from build123d import *

# Parameters (mm, degrees)
CROQUIS1_W              = 5
CROQUIS1_H              = 33
SALIENTE_EXTRUIR1_DEPTH = 3
CROQUIS3_W              = 7
CROQUIS3_H              = 3
SALIENTE_EXTRUIR2_DEPTH = 7
CORTAR_EXTRUIR1_REACH   = 75.478
CROQUIS4_W              = 4.98
CROQUIS4_H              = 6
CROQUIS5_R              = 1
CORTAR_EXTRUIR4_DEPTH   = 15
CORTAR_EXTRUIR5_DEPTH   = 15
CROQUIS8_W              = 2.5
CROQUIS8_H              = 4.326412588
CORTAR_EXTRUIR6_DEPTH   = 10
CORTAR_EXTRUIR7_REACH   = 75.146
CROQUIS9_W              = 1.2
CROQUIS9_H              = 27.63275501


with BuildPart() as part:
    # Croquis1 → Saliente-Extruir1 (new body)
    with BuildSketch(Plane.XY):
        with Locations((-8.507787801, 55.928529755)):
            Rectangle(CROQUIS1_W, CROQUIS1_H)
    extrude(amount=SALIENTE_EXTRUIR1_DEPTH)

    # Croquis3 → Saliente-Extruir2 (add)
    with BuildSketch(Plane.XZ.offset(-39.428529755)):
        with Locations((-8.507787801, 1.5)):
            Rectangle(CROQUIS3_W, CROQUIS3_H)
    extrude(amount=SALIENTE_EXTRUIR2_DEPTH)

    # Croquis4 → Cortar-Extruir1 (cut, up to next)
    with BuildSketch(Plane.XY.offset(3), mode=Mode.PRIVATE) as cortar_extruir1_sk1:
        with Locations((-8.507787801, 35.428529755)):
            Rectangle(CROQUIS4_W, CROQUIS4_H)
    cortar_extruir1_tool1 = extrude(cortar_extruir1_sk1.sketch, amount=-CORTAR_EXTRUIR1_REACH, mode=Mode.PRIVATE) & part.part
    add(cortar_extruir1_tool1.solids().sort_by_distance((-8.507788, 35.42853, 3))[0], mode=Mode.SUBTRACT)

    # Croquis5 → Cortar-Extruir4 (cut)
    with BuildSketch(Plane.ZY.offset(12.007787801)):
        with Locations(Location((1.5, 70.414414657, 0), (0, 0, 270))):
            Circle(CROQUIS5_R)
        with Locations((1.5, 34.917908979)):
            Circle(CROQUIS5_R)
    extrude(amount=-CORTAR_EXTRUIR4_DEPTH, mode=Mode.SUBTRACT)

    # Croquis7 → Cortar-Extruir5 (cut)
    with BuildSketch(Plane.ZY.offset(12.007787801)):
        with BuildLine():
            Line((3, 71.470870039), (3, 72.821585946))
            Line((3, 72.821585946), (0, 72.821585946))
            Line((0, 72.821585946), (0, 71.470870039))
            ThreePointArc((0, 71.470870039), (1.5, 72.091024013), (3, 71.470870039))
        make_face()
        with BuildLine():
            Line((0, 34.344024201), (0, 31.961571753))
            Line((0, 31.961571753), (3, 31.961571753))
            Line((3, 31.961571753), (3, 34.344024201))
            ThreePointArc((3, 34.344024201), (1.5, 33.311875437), (0, 34.344024201))
        make_face()
    extrude(amount=-CORTAR_EXTRUIR5_DEPTH, mode=Mode.SUBTRACT)

    # Croquis8 → Cortar-Extruir6 (cut)
    with BuildSketch(Plane.XY.offset(3)):
        with Locations((-8.507787801, 70.224491059)):
            Rectangle(CROQUIS8_W, CROQUIS8_H)
    extrude(amount=-CORTAR_EXTRUIR6_DEPTH, mode=Mode.SUBTRACT)

    # Croquis9 → Cortar-Extruir7 (cut, up to next)
    with BuildSketch(Plane.XY.offset(3), mode=Mode.PRIVATE) as cortar_extruir7_sk1:
        with Locations((-10.407787801, 53.24490726)):
            Rectangle(CROQUIS9_W, CROQUIS9_H)
    cortar_extruir7_tool1 = extrude(cortar_extruir7_sk1.sketch, amount=-CORTAR_EXTRUIR7_REACH, mode=Mode.PRIVATE) & part.part
    # Croquis9 → Cortar-Extruir7 (cut, up to next)
    with BuildSketch(Plane.XY.offset(3), mode=Mode.PRIVATE) as cortar_extruir7_sk2:
        with Locations((-6.607787801, 53.24490726)):
            Rectangle(CROQUIS9_W, CROQUIS9_H)
    cortar_extruir7_tool2 = extrude(cortar_extruir7_sk2.sketch, amount=-CORTAR_EXTRUIR7_REACH, mode=Mode.PRIVATE) & part.part
    add(cortar_extruir7_tool1.solids().sort_by_distance((-10.407788, 53.244907, 3))[0], mode=Mode.SUBTRACT)
    add(cortar_extruir7_tool2.solids().sort_by_distance((-6.607788, 53.244907, 3))[0], mode=Mode.SUBTRACT)


solid = part.part
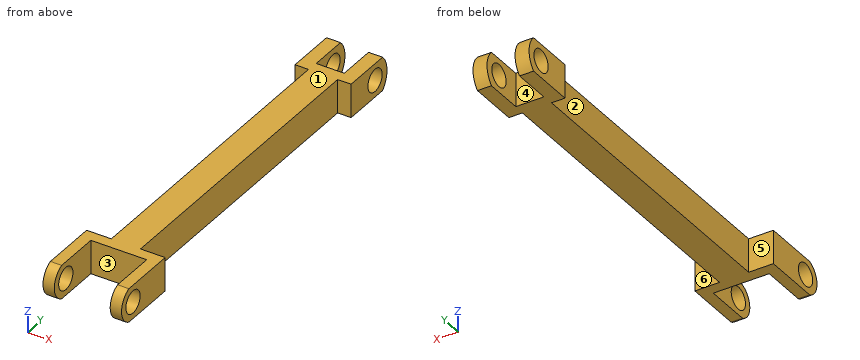
Here's how the part is built. I have some questions about the finished solid (model axes, mm). Face numbers are marked on the shaded views. A direction names the side the tool comes from. Give positions to 0.01 mm unless a question says otherwise; leave off trailing zeros. Write each loop counter-clockwise with the first axis right and the second up, starting at its lowest first coordinate (ties: lowest second). Pieces come first, ordered by that corner, then holes. Notation, with made-up numbers: (-12.5, 57) -> (-5.5, 57) arc R13 cw to (-5.5, 70) -> close; hole circle Ø9 at (11.5, 39). An arc over 180 degrees is marked (long way). Use one line per item in the form item = value. Start each with the question number.
1. Imagine slicing it at B-B on x = -10.5. List the corners of the cut face in (y, z) for me.
2. Imagine slicing it at D-D on x = -5.5. List the corners of the cut face in (y, z) for me.
3. Will these pins go through, and if not, where does the flat tip stop? pin 1 Ø1.3 at (x, z) = (-7, 1) entering from -Y; pin 2 Ø1 at (x, z) = (-8.5, 1.5) entering from +Y; pin 3 Ø1.5 at (y, z) = (69.5, 1) entering from -X.
4. On a 3-axis mill with a long thin cutter (end or side, diameter ignored), from which of +Z, -Z, +X, -X, +Y, -Y can I reach the whole of each face in a straight line? I mean the marked faces 4, 5 and 6. Say none if no direction works.
5. Imagine slicing it at A-A on y = 38. List the corners of the cut face in (x, z) for me.
6. Thinking about a two-plate mould opening in Y: for the marked faces 1, 2 and 3, which applies, +Y half, -Y half, draft (parallel to the pull), parting line (faces both ways), or undercut?
7. If I drill on L1, parallel to X at y = 68.5, z = 0.35; L2, parallel to X at y = 37.5, z = 1.5; L3, parallel to X at y = 46, z = 0.65, over which ranges is the centre line in solid material (lowest first)?
8. Imagine slicing it at C-C on z = 1.5. State how many separate pieces and enclosed holes the cut face has, plus the area to 3 significant figures.
Entries:
q1.outline = (38.43, 0) -> (39.43, 0) -> (39.43, 3) -> (38.43, 3) -> close; (67.06, 0) -> (71.47, 0) arc R2.12 ccw to (71.47, 3) -> (67.06, 3) -> close; hole circle Ø2 at (70.41, 1.5)
q2.outline = (34.34, 0) -> (39.43, 0) -> (39.43, 3) -> (34.34, 3) arc R1.61 ccw to start; hole circle Ø2 at (34.92, 1.5)
q3.pin_1 = 38.43
q3.pin_2 = 68.06
q3.pin_3 = -11.01
q4.face_4 = +Z, -Z, +Y
q4.face_5 = +Z, -Z, -X
q4.face_6 = +Z, -Z, +X
q5.outline = (-12.01, 0) -> (-11, 0) -> (-11, 3) -> (-12.01, 3) -> close; (-6.02, 0) -> (-5.01, 0) -> (-5.01, 3) -> (-6.02, 3) -> close
q6.face_1 = draft
q6.face_2 = undercut
q6.face_3 = -Y half
q7.L1 = -11.01 to -9.76, -7.26 to -6.01
q7.L2 = -12.01 to -11, -6.02 to -5.01
q7.L3 = -9.81 to -7.21
q8.separate_pieces = 5
q8.enclosed_holes = 0
q8.area = 95.2 mm²
